Autodesk Inventor part; units mm, degrees
ref_plane "NUT_ROD_XY" through (0, 0, 0) normal (1, 0, 0) x (0, 0, -1)
ref_plane "NUT_ROD_YZ" through (0, 0, 0) normal (0, 0, -1) x (0, 1, 0)
ref_plane "NUT_ROD_ZX" through (0, 0, 0) normal (0, 1, 0) x (1, 0, 0)
sketch "Sketch_2" plane through (0, 0, 0) normal (0, 0, 1) x (1, 0, 0)
  line L0 (3, 0) -> (-3, 0)
  line L1 (-3, 8) -> (-3, 5)
  line L2 (-3, 5) -> (-2.3235, 4.3235)
  line L3 (-2.3235, 4.3235) -> (2.3235, 4.3235)
  line L4 (2.3235, 4.3235) -> (3, 5)
  line L5 (3, 5) -> (3, 8)
  line L6 (3, 8) -> (1.955, 11.9)
  line L7 (1.955, 11.9) -> (-1.955, 11.9)
  line L8 (-1.955, 11.9) -> (-3, 8)
revolve "Revolution1" add sketch "Sketch_2" angle 360 about axis through (3, 0, 0) along (1, 0, 0)
thread "Thread1"
sketch "Sketch_3" plane through (0, 0, 0) normal (1, 0, 0) x (0, 1, 0)
  circle A0 centre (0, 0) radius 17
  line L0 (-4.9075, 8.5) -> (-9.815, 0)
  line L1 (-9.815, 0) -> (-4.9075, -8.5)
  line L2 (-4.9075, -8.5) -> (4.9075, -8.5)
  line L3 (4.9075, -8.5) -> (9.815, 0)
  line L4 (9.815, 0) -> (4.9075, 8.5)
  line L5 (4.9075, 8.5) -> (-4.9075, 8.5)
extrude "Extrusion1" cut sketch "Sketch_3" along normal mid plane 6
ref_plane "NUT_ROD_XY" through (0, 0, 0) normal (1, 0, 0) x (0, 0, -1)
ref_plane "NUT_ROD_YZ" through (0, 0, 0) normal (0, 0, -1) x (0, 1, 0)
ref_plane "NUT_ROD_ZX" through (0, 0, 0) normal (0, 1, 0) x (1, 0, 0)
properties part number "C96S32_NUT"
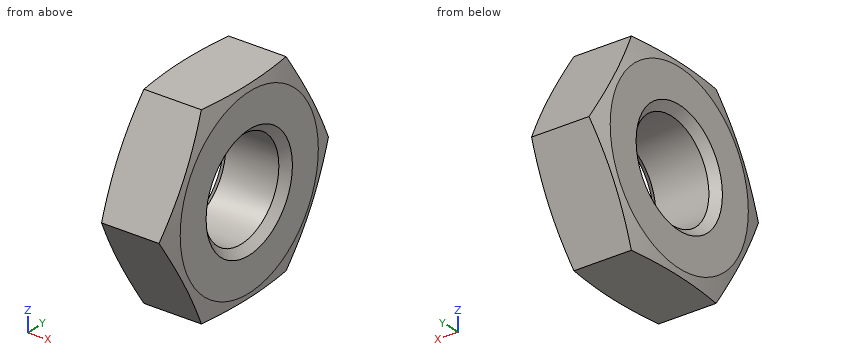
Input: part model. Units: mm. Frame: model coordinates. Give positions to 0.01 mm unless a question says otherwise; leave off trailing zeros. Write each loop counter-clockwise with the first axis right and the second up, starting at its lowest first coordinate (ties: lowest second). Pieces come first, ordered by that corner, then holes.
Q1. Material intervals for probe 1 along Z at (x, y) = (-0.6, 0); probe 2 along Y at (x, z) = (2.1, 0.25); probe 3 along Y at (x, z) = (-0.4, -1.75), sorted ascending.
Q2. First-contact query: P1, Ø2, axis at x = 0, y = -7, coming from the -Z side. Flat tip, straight axial feed; report the tip coordinate or a pass-through.
Q3. Section A-A, the plane y = 0. Output: boundary loops of the cut face in (x, z).
Filled in:
1. probe 1: z = -8.5 to -4.32, 4.32 to 8.5
1. probe 2: y = -9.67 to -4.32, 4.32 to 9.67
1. probe 3: y = -8.8 to -3.95, 3.95 to 8.8
2. P1: stops at z = -6.61
3. outline: (-3, -8) - (-2.87, -8.5) - (2.87, -8.5) - (3, -8) - (3, -5) - (2.32, -4.32) - (-2.32, -4.32) - (-3, -5) - close; (-3, 5) - (-2.32, 4.32) - (2.32, 4.32) - (3, 5) - (3, 8) - (2.87, 8.5) - (-2.87, 8.5) - (-3, 8) - close
